Here's how the part is built. I have some questions about the finished solid (model axes, mm). Round coordinates to 2 decimals unless told otherwise and drop trailing zeros. Order: outer loops, then holes, each group sorted by start corner. A loop starts at its lowest first (then second) coordinate and runs counter-clockwise, first axis right, second up. Notation, with made-up numbers: M 87,-4 L 140,-4 A26 cw 140,26 Z; hole C 86.5,72 d8. An arc over 180 degrees is marked long. Write item = value, one per line. Start each with the question number.
Item 1: Please list where these lines run through material, in increasing order: L1, parallel to Y at x = 0, z = 0; L2, parallel to Y at x = -1.25, z = 0.15; L3, parallel to X at y = -1.25, z = -0.1.
Item 2: I want a section at A-A, the plane y = 0. List the corners of the cut face in (x, z) for me, plus the area to 3 significant figures.
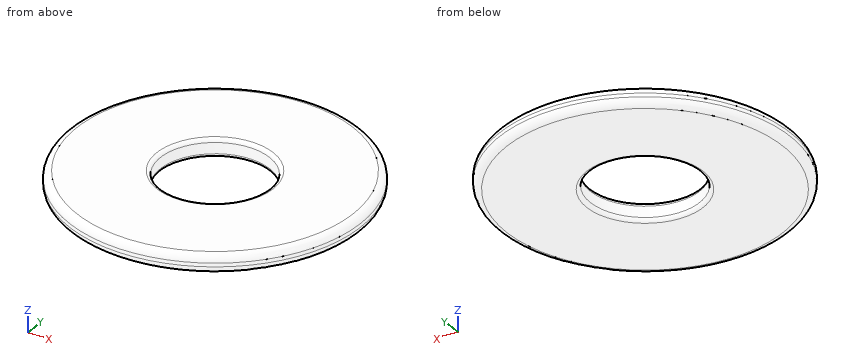
Autodesk Inventor part; units mm, degrees
ref_plane "YZ Plane" through (0, 0, 0) normal (1, 0, 0) x (0, 1, 0)
ref_plane "XZ Plane" through (0, 0, 0) normal (0, 1, 0) x (-1, 0, 0)
ref_plane "XY Plane" through (0, 0, 0) normal (0, 0, 1) x (1, 0, 0)
sketch "Sketch1" plane through (0, 0, 0) normal (0, 0, 1) x (1, 0, 0)
  circle A0 centre (0, 0) radius 1.5
  circle A1 centre (0, 0) radius 4
  dimension "Di" = 3
  dimension "D" = 8
extrude "Extrusion1" add sketch "Sketch1" along normal mid plane 0.5
fillet "Fillet1" radius 0.2 2 edges at (-4, 0, 0.25) (-4, 0, -0.25)
fillet "Fillet2" radius 0.1 2 edges at (-1.5, 0, 0.25) (-1.5, 0, -0.25)
properties part number "Anilha_M3" material "Stainless Steel"
Filled in:
q1.L1 = -4 to -1.5, 1.5 to 4
q1.L2 = -3.77 to -0.83, 0.83 to 3.77
q1.L3 = -3.79 to -0.83, 0.83 to 3.79
q2.outline = M -4,-0.05 A0.2 ccw -3.8,-0.25 L -1.6,-0.25 A0.1 ccw -1.5,-0.15 L -1.5,0.15 A0.1 ccw -1.6,0.25 L -3.8,0.25 A0.2 ccw -4,0.05 Z; M 1.5,-0.15 A0.1 ccw 1.6,-0.25 L 3.8,-0.25 A0.2 ccw 4,-0.05 L 4,0.05 A0.2 ccw 3.8,0.25 L 1.6,0.25 A0.1 ccw 1.5,0.15 Z
q2.area = 2.46 mm^2
